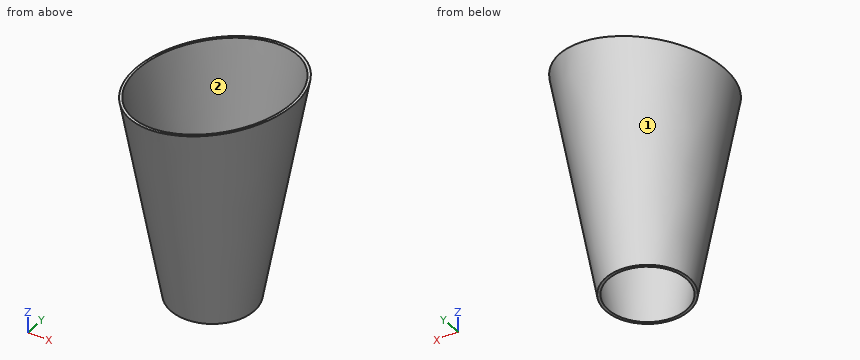
```python
from build123d import *

# Parameters (mm, degrees)
BOX001_W           = 200
BOX001_H           = 199
BOX001_DEPTH       = 200
BOX001_PITCH_ANGLE = -10


with BuildPart() as cube001:
    # Box001 → Box001 (new body)
    with BuildSketch(Plane.XY):
        with Locations((100, 99.5)):
            Rectangle(BOX001_W, BOX001_H)
    extrude(amount=BOX001_DEPTH)


with BuildPart() as cube001_1:
    # Box001 pitch: moved
    add(cube001.part.rotate(Axis((0, 0, 0), (0, 1, 0)), BOX001_PITCH_ANGLE))


with BuildPart() as cube001_2:
    # Box001 placement: moved
    add(cube001_1.part.moved(Location((-95, -94, 142))))


with BuildPart() as center_shade_62mm_base:
    # Sketch001 → Revolution001 (revolve)
    with BuildSketch(Plane.XZ):
        Polygon((31, 0), (60.975587, 170), (58.975587, 170), (29, 0), align=None)
    revolve(axis=Axis((0, 0, 0), (0, 0, 1)))

    # Cut001: cut Cube001
    add(cube001_2.part, mode=Mode.SUBTRACT)


solid = center_shade_62mm_base.part
```
The model under review builds one solid part; all positions refer to its coordinate system, in mm. Face numbers are marked on the shaded views. Round coordinates to 2 decimals unless told otherwise and drop trailing zeros. Write each loop counter-clockwise with the first axis right and the second up, starting at its lowest first coordinate (ties: lowest second). Pieces come first, ordered by that corner, then holes.
(1) Wall thickness on L1, parallel to X at y = -29, z = 23; L2, parallel to X at y = 19, z = 48; L3, parallel to Y at x = 24.5, z = 54: over which ranges is each line inside the solid? List them lowest first.
(2) Insertion check: pin 1 (4 mm diameter, centred on y = -6, z = 75, fed in from -X); pin 2 (4 mm diameter, centred on x = 25.5, z = 20.5, fed in from -Y); pin 3 (4 mm diameter, centred on x = -37.5, z = 134, fed in from -Y). Each pin has a flat end and moves straight along its axis. Give the tip position at first contact, or say it passes through.
(3) We need section A-A on y = 0. Give the boundary of the cut face in (x, z), and give its area (3 significant figures).
(4) We need section D-D on z = 84. Give the boundary of the cut face in (x, y).
(5) We need section B-B on x = 0. Give the boundary of the cut face in (y, z), and give its area (3 significant figures).
(6) We need section C-C on z = 47. Give the boundary of the cut face in (x, y), and give its area (3 significant figures).
(7) Mouldability with a two-part tool opening along Y and no side actions: class the marked faces 1 and 2 as +Y half, -Y half, draft (parallel to the pull), parting line (faces both ways), or undercut.
Findings below:
1. L1: x = -19.69 to -15.86, 15.86 to 19.69
1. L2: x = -34.59 to -32.29, 32.29 to 34.59
1. L3: y = -32.28 to -29.73, 29.73 to 32.28
2. pin 1: stops at x = -44.25
2. pin 2: stops at y = -25.48
2. pin 3: stops at y = -41.58
3. outline: (-57.21, 148.66) - (-31, 0) - (-29, 0) - (-55.27, 149) - close; (29, 0) - (31, 0) - (60.89, 169.49) - (58.82, 169.12) - close
3. area: 636 mm2
4. outline: circle Ø91.62 at (0, 0); hole circle Ø87.62 at (0, 0)
5. outline: (-58.99, 158.75) - (-31, 0) - (-29, 0) - (-56.99, 158.75) - close; (29, 0) - (31, 0) - (58.99, 158.75) - (56.99, 158.75) - close
5. area: 635 mm2
6. outline: circle Ø78.57 at (0, 0); hole circle Ø74.57 at (0, 0)
6. area: 481 mm2
7. face 1: parting line
7. face 2: undercut
